Geometry: final body of the model. Coordinates: model frame, mm. Face numbers are marked on the shaded views. Coordinates: 2 decimals unless noted, no trailing zeros. Loops run counter-clockwise (first coordinate to the right, second up) from the corner with the lowest first, then second, coordinate; pieces in that order, holes last. Notation, with made-up numbers: (40.25, 11.25) -> (65.25, 11.25) arc R32 ccw to (65.25, 38.25) -> close; hole circle Ø9 at (8, 15.25). An arc over 180 degrees is marked (long way). One line per item, written item: value. Start each with the question number.
Item 1: Section query B-B on y = -12.5. Return loops of the section in (x, z), then the cut area to 3 significant figures.
Item 2: Section query A-A on x = 0. Return loops of the section in (y, z).
Item 3: Section query C-C on z = 11.25. Return loops of the section in (x, y).
Item 4: Contact query for flat-ended pins moving along their axis: pin 1 Ø1.6 at (x, y) = (-29, 0.5) entering from +Z (3 decimals); pin 2 Ø4.5 at (x, y) = (29.5, 0) entering from +Z; pin 3 Ø10 at (x, z) = (25.5, 8.5) entering from -Y; pin 4 Ø1 at (x, z) = (25.5, 13.5) entering from -Y. Output: stop coordinate, or through.
Item 5: Mould query, pull axis Y, two halves, no side actions, for the marked faces 1, 2 and 3. Classes: +Y half, -Y half, draft (parallel to the pull), parting line (faces both ways), or undercut.
Item 6: Ray query, probe 1 along Y at (x, z) = (0, 18.65); probe 2 along X at (y, z) = (-22, 18.5); probe 3 along X at (y, z) = (-27.5, 1). Return the intervals inside material, ascending. Write a range as from..to.
Item 7: Section query D-D on x = 13. Return loops of the section in (y, z), then the cut area to 3 significant figures.
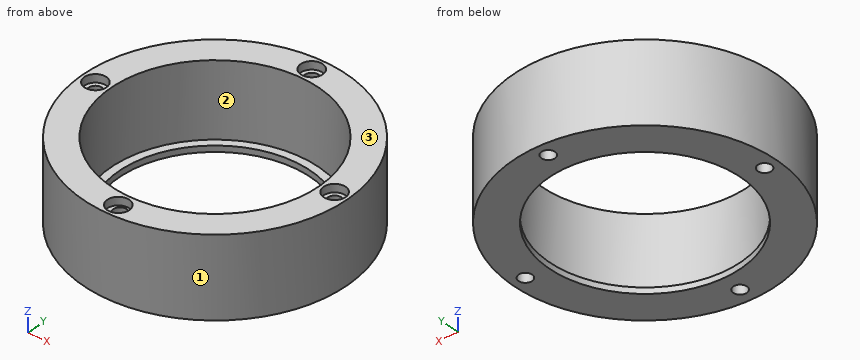
from build123d import *

# Parameters (mm, degrees)
SKETCH1_R           = 33
SKETCH1_R_2         = 24
BOSS_EXTRUDE1_DEPTH = 1.5
SKETCH3_R           = 33
SKETCH3_R_2         = 26
BOSS_EXTRUDE2_DEPTH = 18.5
SKETCH4_R           = 1.7
CUT_EXTRUDE1_DEPTH  = 51.774009099
SKETCH5_R           = 2.75
CUT_EXTRUDE2_DEPTH  = 2


with BuildPart() as part:
    # Sketch1 → Boss-Extrude1 (new body)
    with BuildSketch(Plane.XY):
        Circle(SKETCH1_R)
        Circle(SKETCH1_R_2, mode=Mode.SUBTRACT)
    extrude(amount=BOSS_EXTRUDE1_DEPTH)

    # Sketch3 → Boss-Extrude2 (add)
    with BuildSketch(Plane.XY.offset(1.5)):
        Circle(SKETCH3_R)
        Circle(SKETCH3_R_2, mode=Mode.SUBTRACT)
    extrude(amount=BOSS_EXTRUDE2_DEPTH)

    # Sketch4 → Cut-Extrude1 (cut, through all)
    with BuildSketch(Plane.XY.offset(20)):
        with Locations((0, 29.5)):
            Circle(SKETCH4_R)
        with Locations((29.5, 0)):
            Circle(SKETCH4_R)
        with Locations((0, -29)):
            Circle(SKETCH4_R)
        with Locations((-29.5, 0)):
            Circle(SKETCH4_R)
    extrude(amount=-CUT_EXTRUDE1_DEPTH, mode=Mode.SUBTRACT)

    # Sketch5 → Cut-Extrude2 (cut)
    with BuildSketch(Plane.XY.offset(20)):
        with Locations((0, 29.5)):
            Circle(SKETCH5_R)
        with Locations((29.5, 0)):
            Circle(SKETCH5_R)
        with Locations((0, -29.5)):
            Circle(SKETCH5_R)
        with Locations((-29.5, 0)):
            Circle(SKETCH5_R)
    extrude(amount=-CUT_EXTRUDE2_DEPTH, mode=Mode.SUBTRACT)


solid = part.part
Reply:
1. outline: (-30.54, 0) -> (-20.49, 0) -> (-20.49, 1.5) -> (-22.8, 1.5) -> (-22.8, 20) -> (-30.54, 20) -> close; (20.49, 0) -> (30.54, 0) -> (30.54, 20) -> (22.8, 20) -> (22.8, 1.5) -> (20.49, 1.5) -> close
1. area: 317 mm²
2. outline: (-33, 0) -> (-30.7, 0) -> (-30.7, 18) -> (-32.25, 18) -> (-32.25, 20) -> (-33, 20) -> close; (-27.3, 0) -> (-24, 0) -> (-24, 1.5) -> (-26, 1.5) -> (-26, 20) -> (-26.75, 20) -> (-26.75, 18) -> (-27.3, 18) -> close; (24, 0) -> (27.8, 0) -> (27.8, 18) -> (26.75, 18) -> (26.75, 20) -> (26, 20) -> (26, 1.5) -> (24, 1.5) -> close; (31.2, 0) -> (33, 0) -> (33, 20) -> (32.25, 20) -> (32.25, 18) -> (31.2, 18) -> close
3. outline: circle Ø66 at (0, 0); hole circle Ø3.4 at (-29.5, 0); hole circle Ø52 at (0, 0); hole circle Ø3.4 at (0, -29); hole circle Ø3.4 at (0, 29.5); hole circle Ø3.4 at (29.5, 0)
4. pin 1: passes through
4. pin 2: stops at z = 18
4. pin 3: stops at y = -25.86
4. pin 4: stops at y = -21.54
5. face 1: parting line
5. face 2: undercut
5. face 3: draft
6. probe 1: y = -33..-32.25, -26.75..-26, 26..26.75, 32.25..33
6. probe 2: x = -24.6..-13.86, 13.86..24.6
6. probe 3: x = -18.24..-0.8, 0.8..18.24
7. outline: (-30.33, 0) -> (-20.17, 0) -> (-20.17, 1.5) -> (-22.52, 1.5) -> (-22.52, 20) -> (-30.33, 20) -> close; (20.17, 0) -> (30.33, 0) -> (30.33, 20) -> (22.52, 20) -> (22.52, 1.5) -> (20.17, 1.5) -> close
7. area: 320 mm²
